Check sheet for the modelled part. Datum: model origin and axes. Units: mm. A direction names the side the tool comes from. Round coordinates to 2 decimals unless told otherwise and drop trailing zeros. Loops run counter-clockwise (first coordinate to the right, second up) from the corner with the lowest first, then second, coordinate; pieces in that order, holes last. Notation, with made-up numbers: (-8, 20.25) -> (22, 20.25) arc R13 ccw to (22, 37.25) -> close; hole circle Ø4 at (-7, 52.25). An arc over 180 degrees is marked (long way). One line per item, written item: value. Start each with the question number.
1. Cross-section at A-A on x = 26. Record the cut outline in (y, z).
2. Go/stop test with a flat-tipped pin: pin 1 (1.9 mm diameter, centred on x = 66, z = 41, fed in from +Y). Record where the tip stops, or that it passes through.
3. Set-up check for faces 5 (the face through (-69.85, 25, 1)), 6 (the face through (64, 29.277, 0)), 7 (the face through (-64.15, 44.54, 40.89)): record each of +Z, -Z, +X, -X, +Y, -Y from which the full face is reachable in a straight line by a thin tool's end or side.
4. Cross-section at D-D on x = 66.04. Record the cut outline in (y, z) (3 decimals).
5. Material ranges on L1, parallel to Z at x = -66, y = 44; L2, parallel to X at y = 41.5, z = -40.64 (3 decimals); L3, parallel to X at y = 22, z = -27.5, recorded low to high.
6. Cross-section at C-C on z = -16.5. Record the cut outline in (x, y).
7. Cross-section at B-B on y = 18. Record the cut outline in (x, z), then the cut area to 3 significant figures.
8. Release check for a two-part mould opening along Z. For faces 1 (the face through (-66, 38.1, 41)), 2 (the face through (-1, 25, -44.45)), 3 (the face through (64.15, 44.54, 40.89)), 4 (the face through (-1, 25, 44.45)) record: +Z half, -Z half, draft (parallel to the pull), parting line (faces both ways), or undercut.
from build123d import *

# Parameters (mm, degrees)
SKETCH1_W               = 139.7
SKETCH1_H               = 88.9
BOSS_EXTRUDE1_DEPTH     = 50.8
SKETCH3_W               = 114.3
SKETCH3_H               = 63.5
CUT_EXTRUDE1_DEPTH      = 38.1
SKETCH6_W               = 123.825
SKETCH6_H               = 73.025
SKETCH6_W_2             = 117.475
SKETCH6_H_2             = 66.675
CUT_EXTRUDE2_DEPTH      = 6.35
SKETCH7_R               = 1.905
CUT_EXTRUDE3_DEPTH      = 12.7
MIRROR2_COPY_1_SKETCH_R = 1.905
MIRROR2_COPY_1_DEPTH    = 12.7
CUT_EXTRUDE5_DEPTH      = 12.7


with BuildPart() as part:
    # Sketch1 → Boss-Extrude1 (new body)
    with BuildSketch(Plane(origin=(0, 0, 0), x_dir=(1, 0, 0), z_dir=(0, 1, 0))):
        Rectangle(SKETCH1_W, SKETCH1_H)
    extrude(amount=BOSS_EXTRUDE1_DEPTH)

    # Sketch3 → Cut-Extrude1 (cut)
    with BuildSketch(Plane(origin=(0, 50.8, 0), x_dir=(1, 0, 0), z_dir=(0, 1, 0))):
        Rectangle(SKETCH3_W, SKETCH3_H)
    extrude(amount=-CUT_EXTRUDE1_DEPTH, mode=Mode.SUBTRACT)

    # Sketch6 → Cut-Extrude2 (cut)
    with BuildSketch(Plane(origin=(0, 50.8, 0), x_dir=(1, 0, 0), z_dir=(0, 1, 0))):
        Rectangle(SKETCH6_W, SKETCH6_H)
        Rectangle(SKETCH6_W_2, SKETCH6_H_2, mode=Mode.SUBTRACT)
    extrude(amount=-CUT_EXTRUDE2_DEPTH, mode=Mode.SUBTRACT)

    # Sketch7 → Cut-Extrude3 (cut)
    with BuildSketch(Plane(origin=(0, 50.8, 0), x_dir=(1, 0, 0), z_dir=(0, 1, 0))):
        with Locations(Location((-66.04, 40.64, 0), (0, 0, 270))):
            Circle(SKETCH7_R)
    cut_extrude3 = extrude(amount=-CUT_EXTRUDE3_DEPTH, mode=Mode.SUBTRACT)

    # Mirror1: Cut-Extrude3 across plane
    add(cut_extrude3.mirror(Plane(origin=(0, 0, 0), x_dir=(0, 0, 1), z_dir=(1, 0, 0))), mode=Mode.SUBTRACT)

    # Mirror2: Cut-Extrude3 across plane
    add(cut_extrude3.mirror(Plane.XY), mode=Mode.SUBTRACT)

    # Mirror2 copy 1 sketch → Mirror2 copy 1 (cut)
    with BuildSketch(Plane(origin=(0, 50.8, 0), x_dir=(-1, 0, 0), z_dir=(0, 1, 0))):
        with Locations(Location((-66.04, 40.64, 0), (0, 0, 270))):
            Circle(MIRROR2_COPY_1_SKETCH_R)
    extrude(amount=-MIRROR2_COPY_1_DEPTH, mode=Mode.SUBTRACT)

    # Sketch9 → Cut-Extrude5 (cut)
    with BuildSketch(Plane(origin=(69.85, 0, 0), x_dir=(0, 0, -1), z_dir=(1, 0, 0))):
        with BuildLine():
            Line((-3.175, 22.926701198), (3.175, 22.926701198))
            ThreePointArc((3.175, 22.926701198), (6.35, 26.101701198), (3.175, 29.276701198))
            Line((3.175, 29.276701198), (-3.175, 29.276701198))
            ThreePointArc((-3.175, 29.276701198), (-6.35, 26.101701198), (-3.175, 22.926701198))
        make_face()
    extrude(amount=-CUT_EXTRUDE5_DEPTH, mode=Mode.SUBTRACT)


solid = part.part
Taken from the geometry:
1. outline: (0, -44.45) -> (50.8, -44.45) -> (50.8, -36.51) -> (44.45, -36.51) -> (44.45, -33.34) -> (50.8, -33.34) -> (50.8, -31.75) -> (12.7, -31.75) -> (12.7, 31.75) -> (50.8, 31.75) -> (50.8, 33.34) -> (44.45, 33.34) -> (44.45, 36.51) -> (50.8, 36.51) -> (50.8, 44.45) -> (0, 44.45) -> close
2. pin 1: stops at y = 38.1
3. face 5: +Z, -Z, -X, +Y, -Y
3. face 6: +X
3. face 7: +Y
4. outline: (0, -44.45) -> (50.8, -44.45) -> (50.8, -42.545) -> (38.1, -42.545) -> (38.1, -38.735) -> (50.8, -38.735) -> (50.8, 38.735) -> (38.1, 38.735) -> (38.1, 42.545) -> (50.8, 42.545) -> (50.8, 44.45) -> (0, 44.45) -> close; hole (22.927, -3.175) arc R3.175 ccw to (29.277, -3.175) -> (29.277, 3.175) arc R3.175 ccw to (22.927, 3.175) -> close
5. L1: z = -44.45 to -42.54, -38.74 to 38.74, 42.54 to 44.45
5. L2: x = -69.85 to -67.945, -64.135 to 64.135, 67.945 to 69.85
5. L3: x = -69.85 to -57.15, 57.15 to 69.85
6. outline: (-69.85, 0) -> (69.85, 0) -> (69.85, 50.8) -> (61.91, 50.8) -> (61.91, 44.45) -> (58.74, 44.45) -> (58.74, 50.8) -> (57.15, 50.8) -> (57.15, 12.7) -> (-57.15, 12.7) -> (-57.15, 50.8) -> (-58.74, 50.8) -> (-58.74, 44.45) -> (-61.91, 44.45) -> (-61.91, 50.8) -> (-69.85, 50.8) -> close
7. outline: (-69.85, -44.45) -> (69.85, -44.45) -> (69.85, 44.45) -> (-69.85, 44.45) -> close; hole (-57.15, -31.75) -> (57.15, -31.75) -> (57.15, 31.75) -> (-57.15, 31.75) -> close
7. area: 5,160 mm2
8. face 1: undercut
8. face 2: -Z half
8. face 3: undercut
8. face 4: +Z half
